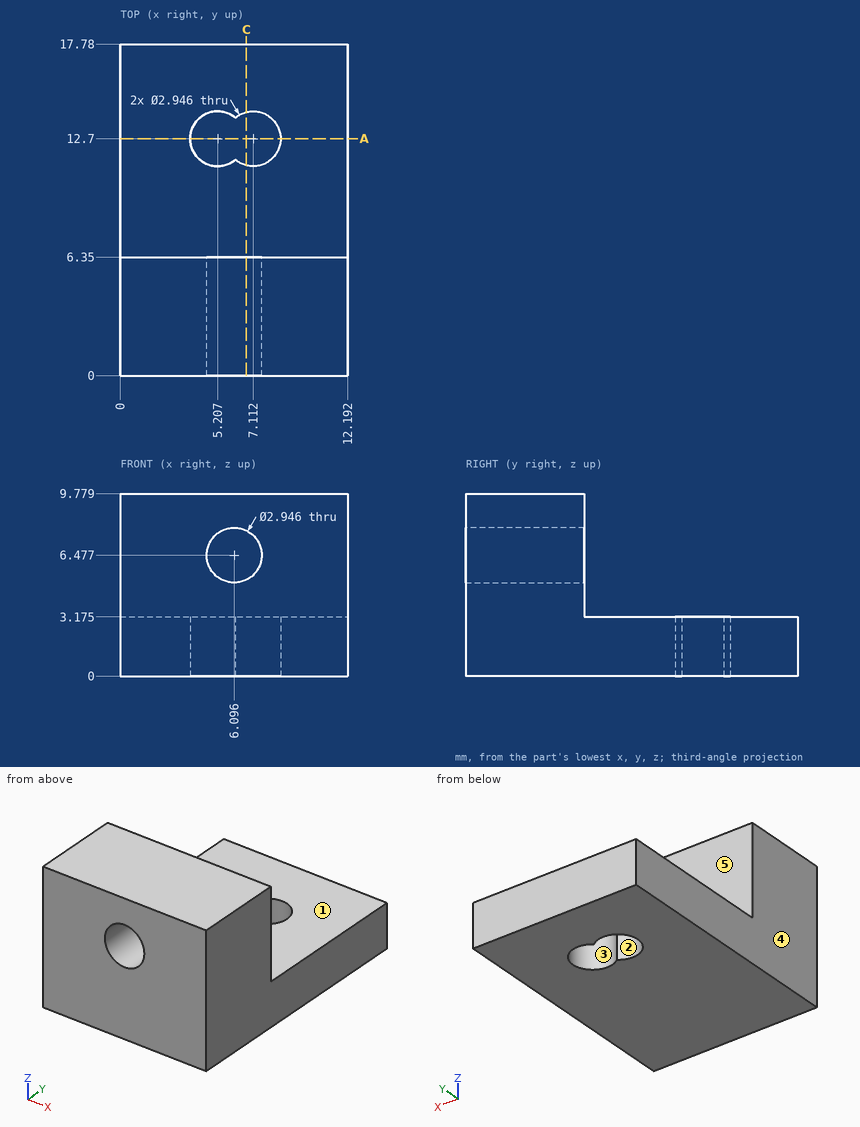
Here's the drawing with two shaded views (mm, measured from the low corner). I have some questions. A direction names the side the tool comes from. Round coordinates to 2 decimals unless told otherwise and drop trailing zeros. Loops run counter-clockwise (first coordinate to the right, second up) from the corner with the lowest first, then second, coordinate; pieces in that order, holes last. Notation, with made-up numbers: (47, 43) - (90, 43) arc R26 ccw to (90, 78) - close; hole circle Ø3 at (5, 25.5). An arc over 180 degrees is marked (long way). Write item = value, one per line.
1) Imagine slicing it at A-A (y = 12.7). Please give me the cut outline in (x, z) (1 decimal), and give its area (3 significant figures).
Computed:
outline = (0, 0) - (3.7, 0) - (3.7, 3.2) - (0, 3.2) - close; (8.6, 0) - (12.2, 0) - (12.2, 3.2) - (8.6, 3.2) - close
area = 23.3 mm2
2) I'm going to push flat-ended pins straight in: P1, Ø2, axis at x = 1.5, y = 8.5, coming from the +Z side (3 decimals); P2, Ø5.5, axis at x = 8.5, z = 6.5, coming from the +Y side; P3, Ø2.5, axis at x = 7.112, y = 12.7, coming from the +Z side. Where does each tip first touch, or does it pass through?
Computed:
P1 = 3.175
P2 = 6.35
P3 = through
3) If we mould it in two halves opening along X, with no side actions, what happens to the marked faces 3, 4 and 5? For each: pulls with the +X half, pulls with the -X half, needs draft (parallel to the pull), parting line crosses it, or undercut.
Computed:
face_3 = undercut
face_4 = pulls with the -X half
face_5 = needs draft
4) On a 3-axis mill with a long thin cutter (end or side, diameter ignored), from which of +Z, -Z, +X, -X, +Y, -Y can I reach the whole of each face in a straight line? I mean the marked faces 1 and 2. Say none if no direction works.
Computed:
face_1 = +Z, +X, -X, +Y
face_2 = +Z, -Z
5) I need wall thicknesses on line 1 along X through (y, z) = (12.7, 1.4) (1 decimal); line 2 along Y through (x, z) = (7, 1.5); line 3 along Z through (x, y) = (1.75, 8.5) (1 decimal). Which ranges of each line are inside material? Lowest first, please. Write a range as from..to.
Computed:
line_1 = 0..3.7, 8.6..12.2
line_2 = 0..11.23, 14.17..17.78
line_3 = 0..3.2
6) Imagine slicing it at C-C (x = 6.75). Give the number of separate pieces and of enclosed holes in the cut face.
Computed:
separate_pieces = 3
enclosed_holes = 0
